```python
from build123d import *

# Parameters (mm, degrees)
F0_R     = 50.8
F1_DEPTH = 6.35
F2_D     = 3.175
F3_D     = 3.175


with BuildPart() as f1:
    # F0 (on Front) → F1 (new body)
    with BuildSketch(Plane.XZ):
        Circle(F0_R)
    extrude(amount=F1_DEPTH)

    # F2 (through all)
    with Locations(Plane(origin=(0, 0, 0), x_dir=(1, 0, 0), z_dir=(0, 1, 0))):
        with Locations((0, 0)):
            Hole(F2_D / 2)

    # F3 (through all)
    with Locations(Plane(origin=(0, 0, 0), x_dir=(1, 0, 0), z_dir=(0, 1, 0))):
        with Locations((0, -25.4), (21.9970452561, 12.7), (-21.9970452561, 12.7)):
            Hole(F3_D / 2)


solid = f1.part
```
Read the model definition and answer for the solid it produces. Units are mm, in the model's axes. Coordinates: 2 decimals unless noted, no trailing zeros. Order: outer loops, then holes, each group sorted by start corner. A loop starts at its lowest first (then second) coordinate and runs counter-clockwise, first axis right, second up. Notation, with made-up numbers: (73, -11.5) - (113, -11.5) arc R18 cw to (113, 16.5) - close; hole circle Ø5 at (56.25, 87). An arc over 180 degrees is marked (long way). Answer as a JSON object with one key per item and string values. Group by question number.
Item 1: Section A-A (x = 0) is taken. Give the vertices of the cut face in (y, z).
Item 2: Flat-ended cylindrical pins translate along their axes: P1, Ø1, axis at x = 32.5, y = -5.5, coming from the -Z side; P2, Ø1.5, axis at x = 32.5, y = -1.5, coming from the -Z side; P3, Ø2, axis at x = -7.5, z = 38, coming from the +Y side; P4, Ø1, axis at x = -12, y = -3, coming from the -Z side. Find the tip coordinate at first contact, or state that the pin passes through.
Item 3: Consider probe 1 along Z at (x, y) = (0, -4.25); probe 2 along X at (y, z) = (-2.5, -12.7); probe 3 along Z at (x, y) = (7, -0.5). Determine where each line is inside the solid, lowest interval first. Write a range as from..to.
Item 4: Section D-D (z = -12.7) is taken. Give the vertices of the cut face in (x, y), plus the area to 3 significant figures.
Item 5: Section C-C (y = -3) is taken. Give the vertices of the cut face in (x, z) (1 decimal).
Item 6: The mould has two halves that part along Y. Classify faces 1 (the face through (11, -6.35, 1)), 2 (the face through (11, 0, 1)), 3 (the face through (-11.012, -3.131, -49.592)): +Y half, -Y half, draft (parallel to the pull), parting line (faces both ways), or undercut.
Item 7: Section B-B (z = 0) is taken. Give the vertices of the cut face in (x, y).
Results are:
{
 "1": {"outline": "(-6.35, -50.8) - (0, -50.8) - (0, -1.59) - (-6.35, -1.59) - close; (-6.35, 1.59) - (0, 1.59) - (0, 23.81) - (-6.35, 23.81) - close; (-6.35, 26.99) - (0, 26.99) - (0, 50.8) - (-6.35, 50.8) - close"},
 "2": {"P1": "stops at z = -39.45", "P2": "stops at z = -39.66", "P3": "stops at y = 0", "P4": "stops at z = -49.48"},
 "3": {"probe 1": "z = -50.8..-1.59, 1.59..23.81, 26.99..50.8", "probe 2": "x = -49.19..-23.58, -20.41..20.41, 23.58..49.19", "probe 3": "z = -50.32..50.32"},
 "4": {"outline": "(-49.19, -6.35) - (-23.58, -6.35) - (-23.58, 0) - (-49.19, 0) - close; (-20.41, -6.35) - (20.41, -6.35) - (20.41, 0) - (-20.41, 0) - close; (23.58, -6.35) - (49.19, -6.35) - (49.19, 0) - (23.58, 0) - close", "area": "584 mm^2"},
 "5": {"outline": "circle Ø101.6 at (0, 0); hole circle Ø3.2 at (-22, -12.7); hole circle Ø3.2 at (0, 0); hole circle Ø3.2 at (0, 25.4); hole circle Ø3.2 at (22, -12.7)"},
 "6": {"face 1": "-Y half", "face 2": "+Y half", "face 3": "draft"},
 "7": {"outline": "(-50.8, -6.35) - (-1.59, -6.35) - (-1.59, 0) - (-50.8, 0) - close; (1.59, -6.35) - (50.8, -6.35) - (50.8, 0) - (1.59, 0) - close"}
}
